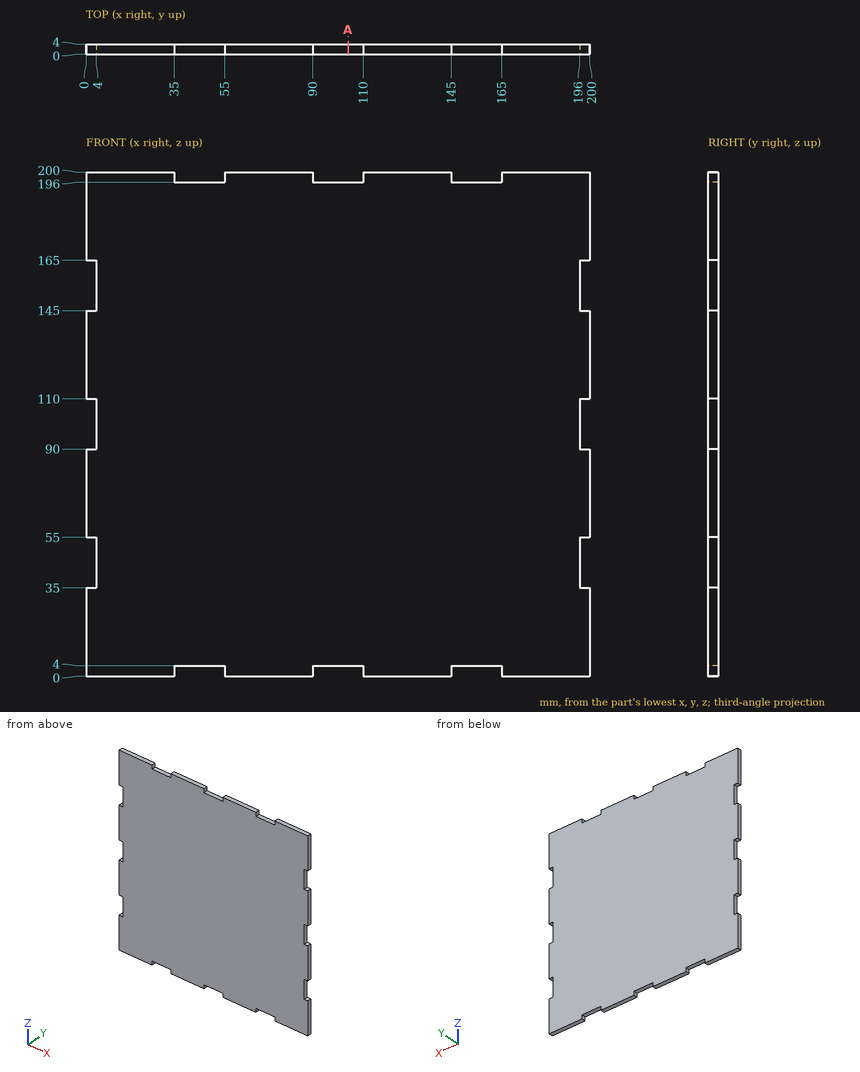
Geometry: see drawing. Coordinates: mm, zero at the bounding-box minimum. Give positions to 0.01 mm unless a question says otherwise; leave off trailing zeros. Loops run counter-clockwise (first coordinate to the right, second up) from the corner with the lowest first, then second, coordinate; pieces in that order, holes last. Notation, with made-up numbers: (-25, -38.75) -> (-8, -38.75) arc R9 ccw to (-8, -30.75) -> close; hole circle Ø8 at (37.25, -3.5). An arc over 180 degrees is marked (long way). Put each result on its own line as item: value.
1. Pin query (flat end, axial travel): P1, Ø1.2, axis at y = 3, z = 157.5, coming from the -X side; P2, Ø1.2, axis at y = 1, z = 98.5, coming from the +X side; P3, Ø2, axis at x = 96, y = 1.5, coming from the -Z side. Return the tip coordinate at first contact, or that it passes through.
Taken from the geometry:
P1: stops at x = 4
P2: stops at x = 196
P3: stops at z = 4
2. Ray query, line 1 along X through (y, z) = (1.9, 97). Return the intervals inside material, ascending. Write a range as [from, to].
Taken from the geometry:
line 1: x = [4, 196]
3. Cut plane A-A (x = 104). Return the cut outline in (y, z).
Taken from the geometry:
outline: (0, 4) -> (4, 4) -> (4, 196) -> (0, 196) -> close
